Autodesk Inventor part; units mm, degrees
ref_plane "ANBAU_XY" through (0, 0, 0) normal (0, 0, 1) x (1, 0, 0)
ref_plane "ANBAU_YZ" through (0, 0, 0) normal (1, 0, 0) x (0, 1, 0)
ref_plane "ANBAU_ZX" through (0, 0, 0) normal (0, 1, 0) x (0, 0, 1)
sketch "Sketch_1" plane through (0, 0, 0) normal (0, 0, 1) x (1, 0, 0)
  arc A0 (-71.5, -61.5) -> (-61.5, -71.5) centre (-61.5, -61.5) ccw
  line L0 (-61.5, -71.5) -> (61.5, -71.5)
  arc A1 (61.5, -71.5) -> (71.5, -61.5) centre (61.5, -61.5) ccw
  line L1 (71.5, -61.5) -> (71.5, 61.5)
  arc A2 (71.5, 61.5) -> (61.5, 71.5) centre (61.5, 61.5) ccw
  line L2 (61.5, 71.5) -> (-61.5, 71.5)
  arc A3 (-61.5, 71.5) -> (-71.5, 61.5) centre (-61.5, 61.5) ccw
  line L3 (-71.5, 61.5) -> (-71.5, -61.5)
  circle A4 centre (58.3363, 58.3363) radius 5.5
  circle A5 centre (58.3363, -58.3363) radius 5.5
  circle A6 centre (-58.3363, 58.3363) radius 5.5
  circle A7 centre (-58.3363, -58.3363) radius 5.5
extrude "Extrusion1" add sketch "Sketch_1" along normal blind 12
sketch "Sketch_2" plane through (0, 0, 0) normal (1, 0, 0) x (0, 1, 0)
  line L0 (0, -3.5) -> (0, 0)
  line L1 (0, 0) -> (65, 0)
  line L2 (65, 0) -> (65, -3.067)
  line L3 (65, -3.067) -> (64.75, -3.5)
  line L4 (64.75, -3.5) -> (0, -3.5)
  line L5 (0, -3.5) -> (0, 0)
revolve "Revolution1" add sketch "Sketch_2" angle 360 about axis through (0, 0, -3.5) along (0, 0, -1)
sketch "Sketch3" plane through (0, 0, -3.5) normal (0, 0, -1) x (-1, 0, 0)
  point P0 (-35.3553, 35.3553)
hole "Hole1" at (35.3553, 35.3553, -3.5) direction (0, 0, 1) diameter 11 depth 15.5
pattern_linear "Rectangular Pattern1" count 2 spacing 70.7107 along (-1, 0, 0) count 2 spacing 70.7107 along (0, -1, 0) of "Hole1"
sketch "Sketch_7" plane through (0, 0, 0) normal (1, 0, 0) x (0, 1, 0)
  line L0 (0, -3.5) -> (0, 12)
  line L1 (0, 12) -> (60.4387, 12)
  arc A0 (60.4387, 12) -> (60.0057, 11.75) centre (60.4387, 11.5) ccw
  line L2 (60.0057, 11.75) -> (59.784, 11.366)
  arc A1 (59.784, 11.366) -> (59.65, 10.866) centre (60.65, 10.866) ccw
  line L3 (59.65, 10.866) -> (59.65, 10.4362)
  arc A2 (59.65, 10.4362) -> (59.6833, 10.1802) centre (60.65, 10.4362) ccw
  arc A3 (59.6572, 7.525) -> (59.6833, 10.1802) centre (54.85, 8.9) ccw
  arc A4 (58.6958, 6.8) -> (59.6572, 7.525) centre (58.6958, 7.8) ccw
  line L4 (58.6958, 6.8) -> (58.15, 6.8)
  line L5 (58.15, 6.8) -> (57.65, 6.3)
  line L6 (57.65, 6.3) -> (57.65, 3)
  line L7 (57.65, 3) -> (40.5, 3)
  line L8 (40.5, 3) -> (40, 2.5)
  line L9 (40, 2.5) -> (40, -3.5)
  line L10 (40, -3.5) -> (0, -3.5)
  line L11 (0, -3.5) -> (0, 12)
revolve "Revolution2" cut sketch "Sketch_7" angle 360 about axis through (0, 0, -3.5) along (0, 0, -1)
sketch "Sketch_16" plane through (0, 0, 0) normal (1, 0, 0) x (0, 1, 0)
  line L0 (0, -2) -> (0, -3.5)
  line L1 (0, -3.5) -> (-60, -3.5)
  line L2 (-60, -3.5) -> (-60, -2)
  line L3 (-60, -2) -> (0, -2)
  line L4 (0, -2) -> (0, -3.5)
revolve "Revolution3" cut sketch "Sketch_16" angle 360 about axis through (0, 0, -2) along (0, 0, 1)
ref_plane "ANBAU_XY" through (0, 0, 0) normal (0, 0, 1) x (1, 0, 0)
ref_plane "ANBAU_YZ" through (0, 0, 0) normal (1, 0, 0) x (0, 1, 0)
ref_plane "ANBAU_ZX" through (0, 0, 0) normal (0, 1, 0) x (0, 0, 1)
ref_plane "M_SCREWS_1_XY" through (-35.3553, -35.3553, -3.5) normal (0, 0, 1) x (1, 0, 0)
ref_plane "M_SCREWS_1_YZ" through (-35.3553, -35.3553, -3.5) normal (1, 0, 0) x (0, 1, 0)
ref_plane "M_SCREWS_1_ZX" through (-35.3553, -35.3553, -3.5) normal (0, 1, 0) x (0, 0, 1)
ref_plane "M_SCREWS_2_XY" through (35.3553, -35.3553, -3.5) normal (0, 0, 1) x (1, 0, 0)
ref_plane "M_SCREWS_2_YZ" through (35.3553, -35.3553, -3.5) normal (1, 0, 0) x (0, 1, 0)
ref_plane "M_SCREWS_2_ZX" through (35.3553, -35.3553, -3.5) normal (0, 1, 0) x (0, 0, 1)
ref_plane "M_SCREWS_3_XY" through (35.3553, 35.3553, -3.5) normal (0, 0, 1) x (1, 0, 0)
ref_plane "M_SCREWS_3_YZ" through (35.3553, 35.3553, -3.5) normal (1, 0, 0) x (0, 1, 0)
ref_plane "M_SCREWS_3_ZX" through (35.3553, 35.3553, -3.5) normal (0, 1, 0) x (0, 0, 1)
ref_plane "M_SCREWS_4_XY" through (-35.3553, 35.3553, -3.5) normal (0, 0, 1) x (1, 0, 0)
ref_plane "M_SCREWS_4_YZ" through (-35.3553, 35.3553, -3.5) normal (1, 0, 0) x (0, 1, 0)
ref_plane "M_SCREWS_4_ZX" through (-35.3553, 35.3553, -3.5) normal (0, 1, 0) x (0, 0, 1)
ref_plane "RS_1_XY" through (58.3363, 58.3363, 12) normal (0, 0, 1) x (1, 0, 0)
ref_plane "RS_1_YZ" through (58.3363, 58.3363, 12) normal (1, 0, 0) x (0, 1, 0)
ref_plane "RS_1_ZX" through (58.3363, 58.3363, 12) normal (0, 1, 0) x (0, 0, 1)
ref_plane "RS_2_XY" through (-58.3363, 58.3363, 12) normal (0, 0, 1) x (1, 0, 0)
ref_plane "RS_2_YZ" through (-58.3363, 58.3363, 12) normal (1, 0, 0) x (0, 1, 0)
ref_plane "RS_2_ZX" through (-58.3363, 58.3363, 12) normal (0, 1, 0) x (0, 0, 1)
ref_plane "RS_3_XY" through (-58.3363, -58.3363, 12) normal (0, 0, 1) x (1, 0, 0)
ref_plane "RS_3_YZ" through (-58.3363, -58.3363, 12) normal (1, 0, 0) x (0, 1, 0)
ref_plane "RS_3_ZX" through (-58.3363, -58.3363, 12) normal (0, 1, 0) x (0, 0, 1)
ref_plane "RS_4_XY" through (58.3363, -58.3363, 12) normal (0, 0, 1) x (1, 0, 0)
ref_plane "RS_4_YZ" through (58.3363, -58.3363, 12) normal (1, 0, 0) x (0, 1, 0)
ref_plane "RS_4_ZX" through (58.3363, -58.3363, 12) normal (0, 1, 0) x (0, 0, 1)
ref_plane "S2_1_XY" through (58.3363, 58.3363, 12) normal (0, 0, -1) x (1, 0, 0)
ref_plane "S2_1_YZ" through (58.3363, 58.3363, 12) normal (1, 0, 0) x (0, -1, 0)
ref_plane "S2_1_ZX" through (58.3363, 58.3363, 12) normal (0, -1, 0) x (0, 0, -1)
ref_plane "S2_2_XY" through (-58.3363, 58.3363, 12) normal (0, 0, -1) x (1, 0, 0)
ref_plane "S2_2_YZ" through (-58.3363, 58.3363, 12) normal (1, 0, 0) x (0, -1, 0)
ref_plane "S2_2_ZX" through (-58.3363, 58.3363, 12) normal (0, -1, 0) x (0, 0, -1)
ref_plane "S2_3_XY" through (-58.3363, -58.3363, 12) normal (0, 0, -1) x (1, 0, 0)
ref_plane "S2_3_YZ" through (-58.3363, -58.3363, 12) normal (1, 0, 0) x (0, -1, 0)
ref_plane "S2_3_ZX" through (-58.3363, -58.3363, 12) normal (0, -1, 0) x (0, 0, -1)
ref_plane "S2_4_XY" through (58.3363, -58.3363, 12) normal (0, 0, -1) x (1, 0, 0)
ref_plane "S2_4_YZ" through (58.3363, -58.3363, 12) normal (1, 0, 0) x (0, -1, 0)
ref_plane "S2_4_ZX" through (58.3363, -58.3363, 12) normal (0, -1, 0) x (0, 0, -1)
properties part number "2683767 EAMF-U-140A-120G-S1---(ADAX)"
Could you check a few things on this model? Use its own coordinates, in mm. A direction names the side the tool comes from. Coordinates: 2 decimals unless noted, no trailing zeros. Return JSON: item names as keys, results as strings.
(1) I'm going to push flat-ended pins straight in: pin 1 (4 mm diameter, centred on x = 51.5, y = 22.5, fed in from +Z); pin 2 (12.5 mm diameter, centred on x = -35.36, y = 35.36, fed in from +Z). Where does each tip first touch, or does it pass through?
Numbers:
{"pin 1": "stops at z = 6.8", "pin 2": "stops at z = 3"}
(2) We'd pull the mould along X, two halves only. Please class faces 4 (the cylindrical face through (-56.28, -12.5, 4.63)), 5 (the flat face through (-38, -17, 3)), 6 (the flat face through (71.5, -1, 6)), 7 (the flat face through (63, 1, 12)): +X half, -X half, draft (parallel to the pull), parting line (faces both ways), or undercut.
Numbers:
{"face 4": "undercut", "face 5": "undercut", "face 6": "+X half", "face 7": "draft"}
(3) I need wall thicknesses on L1, parallel to X at y = 0, z = 5.3; L2, parallel to Z at x = -10, y = 49; L3, parallel to Z at x = 51, y = -59. Which ranges of each line are inside material? Lowest first, please.
Numbers:
{"L1": "x = -71.5 to -57.65, 57.65 to 71.5", "L2": "z = -2 to 3", "L3": "z = 0 to 12"}
(4) Which directions (+Z, -Z, +X, -X, +Y, -Y) give clear straight access to the entire face, cutting with the end or side of a thin tool? Please do faces 1 (the cylindrical face through (2.64, 59.94, -2.74)), 2 (the cylindrical face through (54.3, 54.6, 5.9)), 3 (the cylindrical face through (17.9, 56.9, 10.6)).
Numbers:
{"face 1": "-Z", "face 2": "+Z, -Z", "face 3": "+Z"}
